Part model, mm, in its own coordinate system. Round coordinates to 2 decimals unless told otherwise and drop trailing zeros. Write each loop counter-clockwise with the first axis right and the second up, starting at its lowest first coordinate (ties: lowest second). Pieces come first, ordered by that corner, then holes.
1) Drill centre lines: L1, parallel to X at y = 2.35, z = -38.1; L2, parallel to Z at x = -12.7, y = 2.7; L3, parallel to Z at x = 6, y = 0. Where is each one in solid material? Low to high.
2) Flat gauge pin, fed straight in: pin 1 (8 mm diameter, centred on x = 0.63, z = 60.32, fed in from +Y). Where does the tip first touch, or does it go through?
3) Saw through at A-A on z = -38.1. Write the cut outline in (x, y), and give its area (3 significant figures).
4) Saw through at B-B on x = 12.7. Write the cut outline in (y, z), and give its area (3 significant figures).
```python
from build123d import *

# Parameters (mm, degrees)
BOSS_EXTRUDE1_DEPTH                             = 76.2
BOSS_EXTRUDE1_DEPTH_BACK                        = 76.2
SKETCH3_W                                       = 50.8
SKETCH3_H                                       = 7.9375
M12_CLEARANCE_HOLE2_D                           = 13.5
CSK_FOR_M5_FLAT_HEAD_MACHINE_SCREW1_D           = 5.3
CSK_FOR_M5_FLAT_HEAD_MACHINE_SCREW1_CSINK_D     = 10.4
CSK_FOR_M5_FLAT_HEAD_MACHINE_SCREW1_CSINK_ANGLE = 90
SKETCH26_W                                      = 50.8
SKETCH26_H                                      = 152.4
BOSS_EXTRUDE2_DEPTH                             = 7.9375


with BuildPart() as part:
    # Sketch3 → Boss-Extrude1 (new, two sides: drawn at the far end of the back side and taken through both)
    with BuildSketch(Plane.XY.offset(-BOSS_EXTRUDE1_DEPTH_BACK)):
        Rectangle(SKETCH3_W, SKETCH3_H)
    extrude(amount=BOSS_EXTRUDE1_DEPTH + BOSS_EXTRUDE1_DEPTH_BACK)

    # M12 Clearance Hole2 (through all)
    with Locations(Plane(origin=(0, 3.96875, 0), x_dir=(1, 0, 0), z_dir=(0, 1, 0))):
        with Locations((0.625840615, -60.325)):
            Hole(M12_CLEARANCE_HOLE2_D / 2)

    # CSK for M5 Flat Head Machine Screw1 (through all)
    with Locations(Plane(origin=(0, -3.96875, 0), x_dir=(-1, 0, 0), z_dir=(0, -1, 0))):
        with Locations((-12.7, 38.1), (12.7, 38.1)):
            CounterSinkHole(CSK_FOR_M5_FLAT_HEAD_MACHINE_SCREW1_D / 2, CSK_FOR_M5_FLAT_HEAD_MACHINE_SCREW1_CSINK_D / 2, counter_sink_angle=CSK_FOR_M5_FLAT_HEAD_MACHINE_SCREW1_CSINK_ANGLE)

    # Sketch26 → Boss-Extrude2 (add)
    with BuildSketch(Plane(origin=(0, 3.96875, 0), x_dir=(1, 0, 0), z_dir=(0, 1, 0))):
        with Locations((0, 152.4)):
            Rectangle(SKETCH26_W, SKETCH26_H)
    extrude(amount=-BOSS_EXTRUDE2_DEPTH)


solid = part.part
```
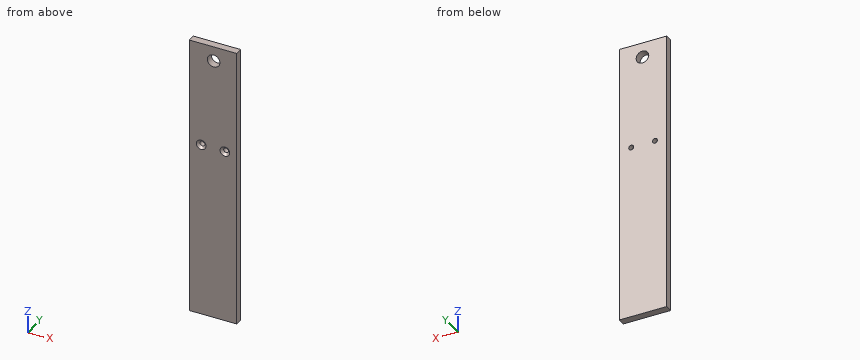
Completed:
1. L1: x = -25.4 to -15.35, -10.05 to 10.05, 15.35 to 25.4
1. L2: z = -228.6 to -40.75, -35.45 to 76.2
1. L3: z = -228.6 to 56.24, 64.41 to 76.2
2. pin 1: passes through
3. outline: (-25.4, -3.97) - (-17.9, -3.97) - (-15.35, -1.42) - (-15.35, 3.97) - (-25.4, 3.97) - close; (-10.05, -1.42) - (-7.5, -3.97) - (7.5, -3.97) - (10.05, -1.42) - (10.05, 3.97) - (-10.05, 3.97) - close; (15.35, -1.42) - (17.9, -3.97) - (25.4, -3.97) - (25.4, 3.97) - (15.35, 3.97) - close
3. area: 306 mm2
4. outline: (-3.97, -228.6) - (3.97, -228.6) - (3.97, -40.75) - (-1.42, -40.75) - (-3.97, -43.3) - close; (-3.97, -32.9) - (-1.42, -35.45) - (3.97, -35.45) - (3.97, 76.2) - (-3.97, 76.2) - close
4. area: 2,370 mm2
